from build123d import *

# Parameters (mm, degrees)
SKETCH1_R          = 3.4
SKETCH1_R_2        = 3.400000006
EXTRUDE1_DEPTH     = 1371.6
SKETCH2_R          = 2.065
CUT_EXTRUDE1_DEPTH = 1373.328945544
SKETCH8_R          = 2.065
CUT_EXTRUDE2_DEPTH = 10


with BuildPart() as part:
    # Sketch1 → Extrude1 (new body)
    with BuildSketch(Plane.XY):
        with BuildLine():
            Line((-36.828217803, 10), (-25.761678346, 10))
            ThreePointArc((-25.761678346, 10), (-24.566343162, 9.581217839), (-24.06, 8.420260776))
            Line((-24.06, 8.420260776), (-24.06, 7.505975062))
            ThreePointArc((-24.06, 7.505975062), (-24.567063435, 6.348506245), (-25.761678346, 5.936507937))
            Line((-25.761678346, 5.936507937), (-26.89856374, 5.936507937))
            Line((-26.89856374, 5.936507937), (-26.89856374, 6.405354551))
            Line((-26.89856374, 6.405354551), (-29.01515873, 6.405354551))
            ThreePointArc((-29.01515873, 6.405354551), (-29.913072103, 6.033426654), (-30.285, 5.135513281))
            Line((-30.285, 5.135513281), (-30.285, 2.878955078))
            ThreePointArc((-30.285, 2.878955078), (-30.217342047, 2.538803338), (-30.024667785, 2.250433031))
            Line((-30.024667785, 2.250433031), (-26.865511635, -0.908897163))
            ThreePointArc((-26.865511635, -0.908897163), (-25.324726136, -1.938463161), (-23.50722312, -2.3))
            Line((-23.50722312, -2.3), (-16.234679932, -2.3))
            ThreePointArc((-16.234679932, -2.3), (-14.417176915, -1.938463161), (-12.876391416, -0.908897163))
            Line((-12.876391416, -0.908897163), (-9.975332215, 1.992321863))
            ThreePointArc((-9.975332215, 1.992321863), (-9.782657953, 2.28069217), (-9.715, 2.620843911))
            Line((-9.715, 2.620843911), (-9.715, 5.135513281))
            ThreePointArc((-9.715, 5.135513281), (-10.086927897, 6.033426654), (-10.98484127, 6.405354551))
            Line((-10.98484127, 6.405354551), (-13.228511431, 6.405354551))
            Line((-13.228511431, 6.405354551), (-13.228511431, 5.936507937))
            Line((-13.228511431, 5.936507937), (-14.365396825, 5.936507937))
            ThreePointArc((-14.365396825, 5.936507937), (-15.478809408, 6.397698529), (-15.94, 7.511111111))
            Line((-15.94, 7.511111111), (-15.94, 8.425396825))
            ThreePointArc((-15.94, 8.425396825), (-15.478809408, 9.538809408), (-14.365396825, 10))
            Line((-14.365396825, 10), (-7.044126982, 10))
            Line((-7.044126982, 10), (14.552471996, 10))
            ThreePointArc((14.552471996, 10), (15.546813416, 9.477564883), (15.94, 8.425396825))
            Line((15.94, 8.425396825), (15.94, 7.511111111))
            ThreePointArc((15.94, 7.511111111), (15.478809408, 6.397698529), (14.365396825, 5.936507937))
            Line((14.365396825, 5.936507937), (13.228511431, 5.936507937))
            Line((13.228511431, 5.936507937), (13.228511431, 6.660633301))
            Line((13.228511431, 6.660633301), (10.98484127, 6.660633301))
            ThreePointArc((10.98484127, 6.660633301), (10.086927897, 6.288705404), (9.715, 5.390792031))
            Line((9.715, 5.390792031), (9.715, 3.134233829))
            ThreePointArc((9.715, 3.134233829), (9.782657953, 2.794082088), (9.975332215, 2.505711781))
            Line((9.975332215, 2.505711781), (13.134488365, -0.653618412))
            ThreePointArc((13.134488365, -0.653618412), (14.64473832, -1.821319739), (16.49277688, -2.3))
            Line((16.49277688, -2.3), (23.50722312, -2.3))
            ThreePointArc((23.50722312, -2.3), (25.324726136, -1.938463161), (26.865511635, -0.908897163))
            Line((26.865511635, -0.908897163), (30.024667785, 2.250433031))
            ThreePointArc((30.024667785, 2.250433031), (30.278278636, 2.655971567), (30.285, 3.134233829))
            Line((30.285, 3.134233829), (30.285, 5.390792031))
            ThreePointArc((30.285, 5.390792031), (29.913072103, 6.288705404), (29.01515873, 6.660633301))
            Line((29.01515873, 6.660633301), (26.771488569, 6.660633301))
            Line((26.771488569, 6.660633301), (26.771488569, 5.936507937))
            Line((26.771488569, 5.936507937), (25.634603175, 5.936507937))
            ThreePointArc((25.634603175, 5.936507937), (24.521190592, 6.397698529), (24.06, 7.511111111))
            Line((24.06, 7.511111111), (24.06, 8.425396825))
            ThreePointArc((24.06, 8.425396825), (24.453186584, 9.477564883), (25.447528004, 10))
            Line((25.447528004, 10), (33.075833554, 10))
            Line((33.075833554, 10), (36.885357363, 10))
            ThreePointArc((36.885357363, 10), (39.090491138, 9.050251023), (40, 6.828217785))
            Line((40, 6.828217785), (40, -6.828217785))
            ThreePointArc((40, -6.828217785), (39.069183486, -9.071177839), (36.825396825, -10))
            Line((36.825396825, -10), (-36.828217803, -10))
            ThreePointArc((-36.828217803, -10), (-39.071006503, -9.071006503), (-40, -6.828217803))
            Line((-40, -6.828217803), (-40, 6.828217803))
            ThreePointArc((-40, 6.828217803), (-39.071006503, 9.071006503), (-36.828217803, 10))
        make_face()
        with Locations((-34.004773868, -4)):
            Circle(SKETCH1_R, mode=Mode.SUBTRACT)
        with Locations(Location((34.004773868, -4, 0), (0, 0, 180))):
            Circle(SKETCH1_R_2, mode=Mode.SUBTRACT)
        with BuildLine():
            Line((-38.35, 2.595292927), (-38.35, 5.557055178))
            ThreePointArc((-38.35, 5.557055178), (-37.509428882, 7.554544736), (-35.493548116, 8.35))
            Line((-35.493548116, 8.35), (-32.569919859, 8.35))
            ThreePointArc((-32.569919859, 8.35), (-32.120963721, 8.164036279), (-31.935, 7.715080141))
            Line((-31.935, 7.715080141), (-31.935, 3.230213422))
            ThreePointArc((-31.935, 3.230213422), (-32.306927856, 2.332300148), (-33.20484113, 1.960372292))
            Line((-33.20484113, 1.960372292), (-37.715079365, 1.960372292))
            ThreePointArc((-37.715079365, 1.960372292), (-38.164036052, 2.14633624), (-38.35, 2.595292927))
        make_face(mode=Mode.SUBTRACT)
        with BuildLine():
            Line((13.450195503, -6.954394873), (-13.450195503, -6.954394873))
            ThreePointArc((-13.450195503, -6.954394873), (-14.036762187, -6.562412722), (-13.89908728, -5.870490687))
            Line((-13.89908728, -5.870490687), (-1.257767926, 6.769315833))
            ThreePointArc((-1.257767926, 6.769315833), (-1.051776589, 6.906937009), (-0.808800063, 6.955252915))
            Line((-0.808800063, 6.955252915), (0, 6.955204454))
            Line((0, 6.955204454), (0.808800063, 6.955252915))
            ThreePointArc((0.808800063, 6.955252915), (1.051776589, 6.906937009), (1.257767926, 6.769315833))
            Line((1.257767926, 6.769315833), (13.89908728, -5.870490687))
            ThreePointArc((13.89908728, -5.870490687), (14.036762187, -6.562412722), (13.450195503, -6.954394873))
        make_face(mode=Mode.SUBTRACT)
        with BuildLine():
            Line((35.554894965, 8.35), (32.563967874, 8.35))
            ThreePointArc((32.563967874, 8.35), (32.121226634, 8.164362109), (31.935, 7.721868186))
            Line((31.935, 7.721868186), (31.935, 3.245873842))
            ThreePointArc((31.935, 3.245873842), (32.306927897, 2.347960469), (33.20484127, 1.976032573))
            Line((33.20484127, 1.976032573), (37.680832198, 1.976032573))
            ThreePointArc((37.680832198, 1.976032573), (38.126707117, 2.122693703), (38.35, 2.535554718))
            Line((38.35, 2.535554718), (38.35, 5.496770698))
            ThreePointArc((38.35, 5.496770698), (37.552616332, 7.511327921), (35.554894965, 8.35))
        make_face(mode=Mode.SUBTRACT)
    extrude(amount=-EXTRUDE1_DEPTH)

    # Sketch2 → Cut-Extrude1 (cut, through all)
    with BuildSketch(Plane.XZ.offset(10)):
        with Locations((-19.935, -1351.6)):
            Circle(SKETCH2_R)
        with Locations((-19.935, -1301.6)):
            Circle(SKETCH2_R)
        with Locations((19.935, -1301.6)):
            Circle(SKETCH2_R)
        with Locations((19.935, -1351.6)):
            Circle(SKETCH2_R)
    extrude(amount=-CUT_EXTRUDE1_DEPTH, mode=Mode.SUBTRACT)

    # Sketch8 → Cut-Extrude2 (cut)
    with BuildSketch(Plane.XZ.offset(10)):
        with Locations((-19.935, -82.4)):
            Circle(SKETCH8_R)
        with Locations((-19.935, -32.4)):
            Circle(SKETCH8_R)
        with Locations((19.935, -32.4)):
            Circle(SKETCH8_R)
        with Locations((19.935, -82.4)):
            Circle(SKETCH8_R)
    extrude(amount=-CUT_EXTRUDE2_DEPTH, mode=Mode.SUBTRACT)


solid = part.part
Design review of the part built by this model. Coordinates are the model's own, in mm. Round coordinates to 2 decimals unless told otherwise and drop trailing zeros. Return JSON: item names as keys, results as strings. Group by question number.
Item 1: The part is to be moulded in two halves that separate along X. For faces 1 (the face through (0, -6.954, -676)), 2 (the face through (1, -10, -676)), say which applies: pulls with the +X half, pulls with the -X half, needs draft (parallel to the pull), parting line crosses it, or undercut.
Item 2: Insertion check: P1, Ø3.5, axis at x = -19.935, z = -1301.6, coming from the -Y side; P2, Ø0.7, axis at y = 8, z = -715, coming from the +X side; P3, Ø5.5, axis at x = 29, z = -722.5, coming from the +Y side; P4, Ø5.5, axis at x = 20, z = -599, coming from the +Y side. Each pin has a flat end and moves straight along its axis. Give the tip position at first contact, or say it passes through.
Item 3: We need section A-A on z = -748. Give the number of separate pieces and of enclosed holes in the cut face, and give its area (3 significant figures).
Item 4: For probe 1 along Y at (x, z) = (-32.5, -695.5); probe 2 along X at (y, z) = (2.25, -1256.5); probe 3 along X at (y, z) = (7.25, -425) (3 decimals), list the stretches that pass through material, from the lowest coordinate up. Write a range as [from, to].
Model answer:
{
 "1": {"face 1": "undercut", "face 2": "needs draft"},
 "2": {"P1": "passes through", "P2": "stops at x = 39.89", "P3": "stops at y = 10", "P4": "stops at y = -2.3"},
 "3": {"separate pieces": "1", "enclosed holes": "5", "area": "851 mm²"},
 "4": {"probe 1": "y = [-10, -7.05], [-0.95, 2.17], [8.35, 10]", "probe 2": "x = [-40, -38.25], [-32.4, -30.02], [-9.8, -5.78], [5.78, 10.23], [30.02, 32.42], [38.24, 40]", "probe 3": "x = [-39.972, -37.779], [-31.935, -24.081], [-15.918, 15.918], [24.082, 31.935], [37.779, 39.972]"}
}
